from build123d import *

# Parameters (mm, degrees)
ESBO_O1_W                = 231.5
ESBO_O1_H                = 96
RESSALTO_EXTRUS_O1_DEPTH = 6
CORTE_EXTRUS_O1_REACH    = 127.451
ESBO_O2_W                = 17.812307692
ESBO_O2_H                = 6
CORTE_EXTRUS_O3_REACH    = 127.451
ESBO_O4_W                = 6
ESBO_O4_H                = 13.715714286
CORTE_EXTRUS_O4_REACH    = 127.451
ESBO_O5_W                = 40
ESBO_O5_H                = 10
CORTE_EXTRUS_O5_REACH    = 127.451
ESBO_O6_W                = 3
ESBO_O6_H                = 10


with BuildPart() as part:
    # Esboço1 → Ressalto-extrusão1 (new body)
    with BuildSketch(Plane.XY):
        Rectangle(ESBO_O1_W, ESBO_O1_H)
    extrude(amount=RESSALTO_EXTRUS_O1_DEPTH)

    # Esboço2 → Corte-extrusão1 (cut, up to next)
    with BuildSketch(Plane(origin=(0, 0, 0), x_dir=(-1, 0, 0), z_dir=(0, 0, -1)), mode=Mode.PRIVATE) as corte_extrus_o1_sk1:
        with Locations((17.796153846, -45)):
            Rectangle(ESBO_O2_W, ESBO_O2_H)
    corte_extrus_o1_tool1 = extrude(corte_extrus_o1_sk1.sketch, amount=-CORTE_EXTRUS_O1_REACH, mode=Mode.PRIVATE) & part.part
    # Esboço2 → Corte-extrusão1 (cut, up to next)
    with BuildSketch(Plane(origin=(0, 0, 0), x_dir=(-1, 0, 0), z_dir=(0, 0, -1)), mode=Mode.PRIVATE) as corte_extrus_o1_sk2:
        with Locations((53.416153846, -45)):
            Rectangle(ESBO_O2_W, ESBO_O2_H)
    corte_extrus_o1_tool2 = extrude(corte_extrus_o1_sk2.sketch, amount=-CORTE_EXTRUS_O1_REACH, mode=Mode.PRIVATE) & part.part
    # Esboço2 → Corte-extrusão1 (cut, up to next)
    with BuildSketch(Plane(origin=(0, 0, 0), x_dir=(-1, 0, 0), z_dir=(0, 0, -1)), mode=Mode.PRIVATE) as corte_extrus_o1_sk3:
        with Locations((89.036153846, -45)):
            Rectangle(ESBO_O2_W, ESBO_O2_H)
    corte_extrus_o1_tool3 = extrude(corte_extrus_o1_sk3.sketch, amount=-CORTE_EXTRUS_O1_REACH, mode=Mode.PRIVATE) & part.part
    # Esboço2 → Corte-extrusão1 (cut, up to next)
    with BuildSketch(Plane(origin=(0, 0, 0), x_dir=(-1, 0, 0), z_dir=(0, 0, -1)), mode=Mode.PRIVATE) as corte_extrus_o1_sk4:
        with Locations((-17.823846154, -45)):
            Rectangle(ESBO_O2_W, ESBO_O2_H)
    corte_extrus_o1_tool4 = extrude(corte_extrus_o1_sk4.sketch, amount=-CORTE_EXTRUS_O1_REACH, mode=Mode.PRIVATE) & part.part
    # Esboço2 → Corte-extrusão1 (cut, up to next)
    with BuildSketch(Plane(origin=(0, 0, 0), x_dir=(-1, 0, 0), z_dir=(0, 0, -1)), mode=Mode.PRIVATE) as corte_extrus_o1_sk5:
        with Locations((-53.443846154, -45)):
            Rectangle(ESBO_O2_W, ESBO_O2_H)
    corte_extrus_o1_tool5 = extrude(corte_extrus_o1_sk5.sketch, amount=-CORTE_EXTRUS_O1_REACH, mode=Mode.PRIVATE) & part.part
    # Esboço2 → Corte-extrusão1 (cut, up to next)
    with BuildSketch(Plane(origin=(0, 0, 0), x_dir=(-1, 0, 0), z_dir=(0, 0, -1)), mode=Mode.PRIVATE) as corte_extrus_o1_sk6:
        with Locations((-89.063846154, -45)):
            Rectangle(ESBO_O2_W, ESBO_O2_H)
    corte_extrus_o1_tool6 = extrude(corte_extrus_o1_sk6.sketch, amount=-CORTE_EXTRUS_O1_REACH, mode=Mode.PRIVATE) & part.part
    # Esboço2 → Corte-extrusão1 (cut, up to next)
    with BuildSketch(Plane(origin=(0, 0, 0), x_dir=(-1, 0, 0), z_dir=(0, 0, -1)), mode=Mode.PRIVATE) as corte_extrus_o1_sk7:
        with Locations((-89.063846154, 48)):
            Rectangle(ESBO_O2_W, ESBO_O2_H)
    corte_extrus_o1_tool7 = extrude(corte_extrus_o1_sk7.sketch, amount=-CORTE_EXTRUS_O1_REACH, mode=Mode.PRIVATE) & part.part
    # Esboço2 → Corte-extrusão1 (cut, up to next)
    with BuildSketch(Plane(origin=(0, 0, 0), x_dir=(-1, 0, 0), z_dir=(0, 0, -1)), mode=Mode.PRIVATE) as corte_extrus_o1_sk8:
        with Locations((-53.443846154, 48)):
            Rectangle(ESBO_O2_W, ESBO_O2_H)
    corte_extrus_o1_tool8 = extrude(corte_extrus_o1_sk8.sketch, amount=-CORTE_EXTRUS_O1_REACH, mode=Mode.PRIVATE) & part.part
    # Esboço2 → Corte-extrusão1 (cut, up to next)
    with BuildSketch(Plane(origin=(0, 0, 0), x_dir=(-1, 0, 0), z_dir=(0, 0, -1)), mode=Mode.PRIVATE) as corte_extrus_o1_sk9:
        with Locations((-17.823846154, 48)):
            Rectangle(ESBO_O2_W, ESBO_O2_H)
    corte_extrus_o1_tool9 = extrude(corte_extrus_o1_sk9.sketch, amount=-CORTE_EXTRUS_O1_REACH, mode=Mode.PRIVATE) & part.part
    # Esboço2 → Corte-extrusão1 (cut, up to next)
    with BuildSketch(Plane(origin=(0, 0, 0), x_dir=(-1, 0, 0), z_dir=(0, 0, -1)), mode=Mode.PRIVATE) as corte_extrus_o1_sk10:
        with Locations((17.796153846, 48)):
            Rectangle(ESBO_O2_W, ESBO_O2_H)
    corte_extrus_o1_tool10 = extrude(corte_extrus_o1_sk10.sketch, amount=-CORTE_EXTRUS_O1_REACH, mode=Mode.PRIVATE) & part.part
    # Esboço2 → Corte-extrusão1 (cut, up to next)
    with BuildSketch(Plane(origin=(0, 0, 0), x_dir=(-1, 0, 0), z_dir=(0, 0, -1)), mode=Mode.PRIVATE) as corte_extrus_o1_sk11:
        with Locations((89.036153846, 48)):
            Rectangle(ESBO_O2_W, ESBO_O2_H)
    corte_extrus_o1_tool11 = extrude(corte_extrus_o1_sk11.sketch, amount=-CORTE_EXTRUS_O1_REACH, mode=Mode.PRIVATE) & part.part
    # Esboço2 → Corte-extrusão1 (cut, up to next)
    with BuildSketch(Plane(origin=(0, 0, 0), x_dir=(-1, 0, 0), z_dir=(0, 0, -1)), mode=Mode.PRIVATE) as corte_extrus_o1_sk12:
        with Locations((53.416153846, 48)):
            Rectangle(ESBO_O2_W, ESBO_O2_H)
    corte_extrus_o1_tool12 = extrude(corte_extrus_o1_sk12.sketch, amount=-CORTE_EXTRUS_O1_REACH, mode=Mode.PRIVATE) & part.part
    add(corte_extrus_o1_tool1.solids().sort_by_distance((-17.796154, -45, 0))[0], mode=Mode.SUBTRACT)
    add(corte_extrus_o1_tool2.solids().sort_by_distance((-53.416154, -45, 0))[0], mode=Mode.SUBTRACT)
    add(corte_extrus_o1_tool3.solids().sort_by_distance((-89.036154, -45, 0))[0], mode=Mode.SUBTRACT)
    add(corte_extrus_o1_tool4.solids().sort_by_distance((17.823846, -45, 0))[0], mode=Mode.SUBTRACT)
    add(corte_extrus_o1_tool5.solids().sort_by_distance((53.443846, -45, 0))[0], mode=Mode.SUBTRACT)
    add(corte_extrus_o1_tool6.solids().sort_by_distance((89.063846, -45, 0))[0], mode=Mode.SUBTRACT)
    add(corte_extrus_o1_tool7.solids().sort_by_distance((89.063846, 48, 0))[0], mode=Mode.SUBTRACT)
    add(corte_extrus_o1_tool8.solids().sort_by_distance((53.443846, 48, 0))[0], mode=Mode.SUBTRACT)
    add(corte_extrus_o1_tool9.solids().sort_by_distance((17.823846, 48, 0))[0], mode=Mode.SUBTRACT)
    add(corte_extrus_o1_tool10.solids().sort_by_distance((-17.796154, 48, 0))[0], mode=Mode.SUBTRACT)
    add(corte_extrus_o1_tool11.solids().sort_by_distance((-89.036154, 48, 0))[0], mode=Mode.SUBTRACT)
    add(corte_extrus_o1_tool12.solids().sort_by_distance((-53.416154, 48, 0))[0], mode=Mode.SUBTRACT)

    # Esboço4 → Corte-extrusão3 (cut, up to next)
    with BuildSketch(Plane(origin=(0, 0, 0), x_dir=(-1, 0, 0), z_dir=(0, 0, -1)), mode=Mode.PRIVATE) as corte_extrus_o3_sk1:
        with Locations((112.75, -0.002142857)):
            Rectangle(ESBO_O4_W, ESBO_O4_H)
    corte_extrus_o3_tool1 = extrude(corte_extrus_o3_sk1.sketch, amount=-CORTE_EXTRUS_O3_REACH, mode=Mode.PRIVATE) & part.part
    # Esboço4 → Corte-extrusão3 (cut, up to next)
    with BuildSketch(Plane(origin=(0, 0, 0), x_dir=(-1, 0, 0), z_dir=(0, 0, -1)), mode=Mode.PRIVATE) as corte_extrus_o3_sk2:
        with Locations((112.75, 27.427857143)):
            Rectangle(ESBO_O4_W, ESBO_O4_H)
    corte_extrus_o3_tool2 = extrude(corte_extrus_o3_sk2.sketch, amount=-CORTE_EXTRUS_O3_REACH, mode=Mode.PRIVATE) & part.part
    # Esboço4 → Corte-extrusão3 (cut, up to next)
    with BuildSketch(Plane(origin=(0, 0, 0), x_dir=(-1, 0, 0), z_dir=(0, 0, -1)), mode=Mode.PRIVATE) as corte_extrus_o3_sk3:
        with Locations((-112.75, 27.427857143)):
            Rectangle(ESBO_O4_W, ESBO_O4_H)
    corte_extrus_o3_tool3 = extrude(corte_extrus_o3_sk3.sketch, amount=-CORTE_EXTRUS_O3_REACH, mode=Mode.PRIVATE) & part.part
    # Esboço4 → Corte-extrusão3 (cut, up to next)
    with BuildSketch(Plane(origin=(0, 0, 0), x_dir=(-1, 0, 0), z_dir=(0, 0, -1)), mode=Mode.PRIVATE) as corte_extrus_o3_sk4:
        with Locations((-112.75, -0.002142857)):
            Rectangle(ESBO_O4_W, ESBO_O4_H)
    corte_extrus_o3_tool4 = extrude(corte_extrus_o3_sk4.sketch, amount=-CORTE_EXTRUS_O3_REACH, mode=Mode.PRIVATE) & part.part
    # Esboço4 → Corte-extrusão3 (cut, up to next)
    with BuildSketch(Plane(origin=(0, 0, 0), x_dir=(-1, 0, 0), z_dir=(0, 0, -1)), mode=Mode.PRIVATE) as corte_extrus_o3_sk5:
        with Locations((-112.75, -27.432142857)):
            Rectangle(ESBO_O4_W, ESBO_O4_H)
    corte_extrus_o3_tool5 = extrude(corte_extrus_o3_sk5.sketch, amount=-CORTE_EXTRUS_O3_REACH, mode=Mode.PRIVATE) & part.part
    # Esboço4 → Corte-extrusão3 (cut, up to next)
    with BuildSketch(Plane(origin=(0, 0, 0), x_dir=(-1, 0, 0), z_dir=(0, 0, -1)), mode=Mode.PRIVATE) as corte_extrus_o3_sk6:
        with Locations((112.75, -27.432142857)):
            Rectangle(ESBO_O4_W, ESBO_O4_H)
    corte_extrus_o3_tool6 = extrude(corte_extrus_o3_sk6.sketch, amount=-CORTE_EXTRUS_O3_REACH, mode=Mode.PRIVATE) & part.part
    add(corte_extrus_o3_tool1.solids().sort_by_distance((-112.75, -0.002143, 0))[0], mode=Mode.SUBTRACT)
    add(corte_extrus_o3_tool2.solids().sort_by_distance((-112.75, 27.427857, 0))[0], mode=Mode.SUBTRACT)
    add(corte_extrus_o3_tool3.solids().sort_by_distance((112.75, 27.427857, 0))[0], mode=Mode.SUBTRACT)
    add(corte_extrus_o3_tool4.solids().sort_by_distance((112.75, -0.002143, 0))[0], mode=Mode.SUBTRACT)
    add(corte_extrus_o3_tool5.solids().sort_by_distance((112.75, -27.432143, 0))[0], mode=Mode.SUBTRACT)
    add(corte_extrus_o3_tool6.solids().sort_by_distance((-112.75, -27.432143, 0))[0], mode=Mode.SUBTRACT)

    # Esboço5 → Corte-extrusão4 (cut, up to next)
    with BuildSketch(Plane(origin=(0, 0, 0), x_dir=(-1, 0, 0), z_dir=(0, 0, -1)), mode=Mode.PRIVATE) as corte_extrus_o4_sk1:
        with Locations((0, 23)):
            Rectangle(ESBO_O5_W, ESBO_O5_H)
    corte_extrus_o4_tool1 = extrude(corte_extrus_o4_sk1.sketch, amount=-CORTE_EXTRUS_O4_REACH, mode=Mode.PRIVATE) & part.part
    add(corte_extrus_o4_tool1.solids().sort_by_distance((0, 23, 0))[0], mode=Mode.SUBTRACT)

    # Esboço6 → Corte-extrusão5 (cut, up to next)
    with BuildSketch(Plane(origin=(0, 0, 0), x_dir=(-1, 0, 0), z_dir=(0, 0, -1)), mode=Mode.PRIVATE) as corte_extrus_o5_sk1:
        with Locations((47, 23)):
            Rectangle(ESBO_O6_W, ESBO_O6_H)
    corte_extrus_o5_tool1 = extrude(corte_extrus_o5_sk1.sketch, amount=-CORTE_EXTRUS_O5_REACH, mode=Mode.PRIVATE) & part.part
    # Esboço6 → Corte-extrusão5 (cut, up to next)
    with BuildSketch(Plane(origin=(0, 0, 0), x_dir=(-1, 0, 0), z_dir=(0, 0, -1)), mode=Mode.PRIVATE) as corte_extrus_o5_sk2:
        with Locations((-47, 23)):
            Rectangle(ESBO_O6_W, ESBO_O6_H)
    corte_extrus_o5_tool2 = extrude(corte_extrus_o5_sk2.sketch, amount=-CORTE_EXTRUS_O5_REACH, mode=Mode.PRIVATE) & part.part
    # Esboço6 → Corte-extrusão5 (cut, up to next)
    with BuildSketch(Plane(origin=(0, 0, 0), x_dir=(-1, 0, 0), z_dir=(0, 0, -1)), mode=Mode.PRIVATE) as corte_extrus_o5_sk3:
        with Locations((-47, 3)):
            Rectangle(ESBO_O6_W, ESBO_O6_H)
    corte_extrus_o5_tool3 = extrude(corte_extrus_o5_sk3.sketch, amount=-CORTE_EXTRUS_O5_REACH, mode=Mode.PRIVATE) & part.part
    # Esboço6 → Corte-extrusão5 (cut, up to next)
    with BuildSketch(Plane(origin=(0, 0, 0), x_dir=(-1, 0, 0), z_dir=(0, 0, -1)), mode=Mode.PRIVATE) as corte_extrus_o5_sk4:
        with Locations((47, 3)):
            Rectangle(ESBO_O6_W, ESBO_O6_H)
    corte_extrus_o5_tool4 = extrude(corte_extrus_o5_sk4.sketch, amount=-CORTE_EXTRUS_O5_REACH, mode=Mode.PRIVATE) & part.part
    add(corte_extrus_o5_tool1.solids().sort_by_distance((-47, 23, 0))[0], mode=Mode.SUBTRACT)
    add(corte_extrus_o5_tool2.solids().sort_by_distance((47, 23, 0))[0], mode=Mode.SUBTRACT)
    add(corte_extrus_o5_tool3.solids().sort_by_distance((47, 3, 0))[0], mode=Mode.SUBTRACT)
    add(corte_extrus_o5_tool4.solids().sort_by_distance((-47, 3, 0))[0], mode=Mode.SUBTRACT)


solid = part.part
The listing builds one solid part. Answer for the finished solid, in the listing's coordinates (mm). A direction names the side the tool comes from. Round coordinates to 2 decimals unless told otherwise and drop trailing zeros. Order: outer loops, then holes, each group sorted by start corner. A loop starts at its lowest first (then second) coordinate and runs counter-clockwise, first axis right, second up. Notation, with made-up numbers: M -35.75,-3 L 22.25,-3 A8 ccw 22.25,5 Z; hole C 7.25,-29 d5. An arc over 180 degrees is marked long. Answer in a Markdown table with one row per item. Add a question column.
1) Which of the six approach directions +Z, -Z, +X, -X, +Y, -Y give full straight-line access (tool end or side, diameter ignored) to faces 1 (the face through (44.538, -45, 3)), 2 (the face through (-48.5, 23, 3)), 3 (the face through (-2, 1, 0)), 4 (the face through (-113, -20.574, 3)), 5 (the face through (113, -20.574, 3))?
2) The part is cut by section A-A on y = 23.5. Determine the outline of the cut face in (x, z).
3) Determine the mould class of faces 6 (the face through (113, 20.57, 3)), 7 (the face through (113, -34.29, 3)), 8 (the face through (-8.89, -45, 3)), 9 (the face through (-107, -48, 3)) for opening direction Y: pulls with the +Y half, pulls with the -Y half, needs draft (parallel to the pull), parting line crosses it, or undercut.
4) The part is cut by section C-C on x = 56.5. Determine the outline of the cut face in (y, z).
5) Flat-ended cylindrical pins translate along their axes: pin 1 Ø1.8 at (x, z) = (14, 2) entering from +Y; pin 2 Ø1.8 at (y, z) = (23.5, 4) entering from -X; pin 3 Ø3 at (y, z) = (2.5, 4) entering from +X; pin 4 Ø3 at (y, z) = (22, 2) entering from -X. Find the tip coordinate at first contact, or state that the pin passes through.
6) Consider line 1 along X through (y, z) = (-0.5, 5.7); line 2 along Y through (x, z) = (-16.5, 1.75); line 3 along Y through (x, z) = (4.5, 1.3). Determine where each line is inside the solid, lowest interval first. Write a range as from..to.
7) The part is cut by section B-B on z = 4.95. Count the separate pieces of the cut face and the enclosed holes in it, plus the area to 3 significant figures.
Findings below:
| question | item | result |
|---|---|---|
| 1 | face 1 | +Z, -Z, -Y |
| 1 | face 2 | +Z, -Z |
| 1 | face 3 | -Z, +X, -X, +Y, -Y |
| 1 | face 4 | +Z, -Z, -X |
| 1 | face 5 | +Z, -Z, +X |
| 2 | outline | M -109.75,0 L -48.5,0 L -48.5,6 L -109.75,6 Z; M -45.5,0 L -20,0 L -20,6 L -45.5,6 Z; M 20,0 L 45.5,0 L 45.5,6 L 20,6 Z; M 48.5,0 L 109.75,0 L 109.75,6 L 48.5,6 Z |
| 3 | face 6 | undercut |
| 3 | face 7 | undercut |
| 3 | face 8 | needs draft |
| 3 | face 9 | pulls with the -Y half |
| 4 | outline | M -42,0 L 45,0 L 45,6 L -42,6 Z |
| 5 | pin 1 | stops at y = 45 |
| 5 | pin 2 | stops at x = -109.75 |
| 5 | pin 3 | stops at x = 109.75 |
| 5 | pin 4 | stops at x = -115.75 |
| 6 | line 1 | x = -109.75..-48.5, -45.5..45.5, 48.5..109.75 |
| 6 | line 2 | y = -42..18, 28..45 |
| 6 | line 3 | y = -48..18, 28..48 |
| 7 | separate pieces | 1 |
| 7 | enclosed holes | 5 |
| 7 | area | 20,200 mm² |
